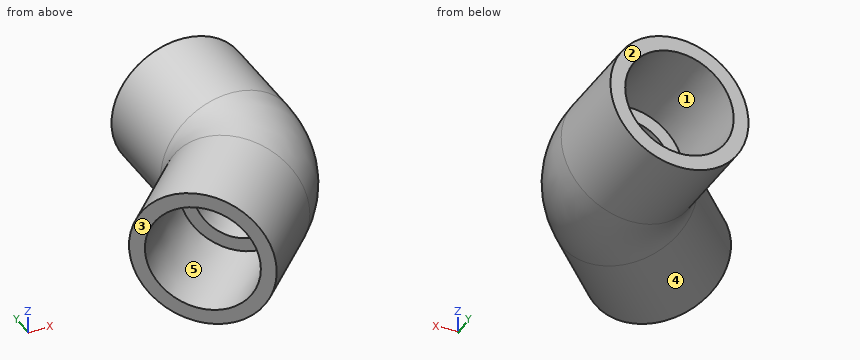
```python
from build123d import *

# Parameters (mm, degrees)
SKETCH3_R   = 13.716
SKETCH3_R_2 = 7.8994


with BuildPart() as part:
    # Sketch1 → Revolve1 (revolve)
    with BuildSketch(Plane.XY):
        Polygon((-8.980256121, -28.377609343), (4.490128061, -14.907225161), (2.298945567, -12.716042667), (-11.063675541, -26.294189922), align=None)
    revolve(axis=Axis((-18.678932732, -18.678932732, 0), (0.707106781, 0.707106781, 0)))



with BuildPart() as body_2:
    # Sketch2 → Revolve2 (revolve)
    with BuildSketch(Plane.XY):
        Polygon((10.7696, 26.416), (10.6172, 7.366), (13.716, 7.366), (13.716, 26.416), align=None)
    revolve(axis=Axis((0, 0, 0), (0, 1, 0)))


with BuildPart() as part_1:
    add(part.part)

    add(body_2.part)  # Sweep1 merges body 2
    # Sweep1: sweep along a path in Sketch4
    with BuildLine(Plane.XY) as sweep1_path:
        ThreePointArc((-5.20854855, -5.20854855), (-1.353657665, 0.560703364), (0, 7.366))
    # Sketch3 → Sweep1 (sweep)
    with BuildSketch(Plane(origin=(-5.20854855, -5.20854855, 0), x_dir=(0, 0, -1), z_dir=(0.707106781, 0.707106781, 0))):
        Circle(SKETCH3_R)
        Circle(SKETCH3_R_2, mode=Mode.SUBTRACT)
    sweep(path=sweep1_path.line)


solid = part_1.part
```
Geometry: final body of the model. Coordinates: model frame, mm. Face numbers are marked on the shaded views. A direction names the side the tool comes from. Coordinates: 2 decimals unless noted, no trailing zeros. Order: outer loops, then holes, each group sorted by start corner. A loop starts at its lowest first (then second) coordinate and runs counter-clockwise, first axis right, second up. Notation, with made-up numbers: (11, 84) -> (70, 84) arc R32 ccw to (70, 114) -> close; hole circle Ø1 at (26.25, 13). An arc over 180 degrees is marked (long way). Answer in a Markdown table with one row per item.
Item 1: Ray query, L1, parallel to Y at x = -9, z = 5.5; L2, parallel to Z at x = -13.5, y = -13.5; L3, parallel to X at y = -8.5, z = 5. Return the intervals inside material, ascending.
Return value:
| item | result |
|---|---|
| L1 | y = -26.77 to -22.04, -0.98 to 7.37 |
| L2 | z = -13.72 to -10.71, 10.71 to 13.72 |
| L3 | x = -26.56 to -21.93, 0.09 to 8.33 |
Item 2: Draft query along Z for the marked faces 3, 4 and 5. Return one class per face: released by +Z, released by -Z, zero draft, split by the parting line, or undercut.
Return value:
| item | result |
|---|---|
| face 3 | zero draft |
| face 4 | split by the parting line |
| face 5 | undercut |
Item 3: Section B-B on y = 16. Output: boundary loops of the cut face in (x, z).
Return value:
| item | result |
|---|---|
| outline | circle Ø27.43 at (0, 0); hole circle Ø21.37 at (0, 0) |
Item 4: Access query for the marked faces 1 and 2. Directions: +Z, -Z, +X, -X, +Y, -Y. A direction counts if a zero-diameter tool reaches every point of the face in a straight line with its end or side. Return the directions, or none.
Return value:
| item | result |
|---|---|
| face 1 | +Y |
| face 2 | +Z, -Z, +X, -X, +Y |
Item 5: Contact query for flat-ended pins moving along their axis: P1, Ø4, axis at x = -15, z = -10.5, coming from the -Y side; P2, Ø5, axis at x = 8.5, y = 17, coming from the +Z side; P3, Ø3, axis at y = 2, z = -3.5, coming from the -X side. Output: stop coordinate, or through.
Return value:
| item | result |
|---|---|
| P1 | stops at y = -24.36 |
| P2 | stops at z = 12.33 |
| P3 | stops at x = -18.34 |
Item 6: Section A-A on z = 12.25. Output: boundary loops of the cut face in (x, y).
Return value:
| item | result |
|---|---|
| outline | (-23.04, -14.32) -> (-14.32, -23.04) -> (-0.85, -9.57) arc R23.95 ccw to (6.17, 7.37) -> (6.17, 26.42) -> (-6.17, 26.42) -> (-6.17, 7.37) arc R11.61 cw to (-9.57, -0.85) -> close |
